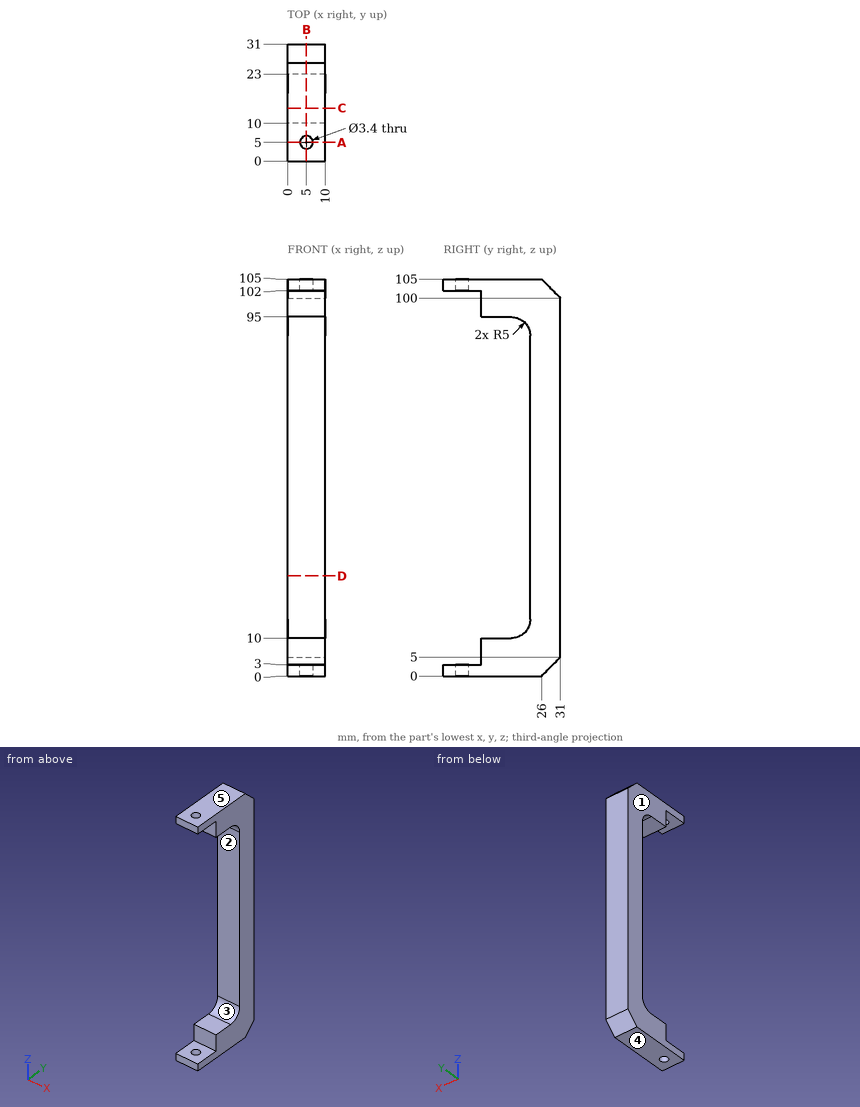
Print and shaded views of the part. All mm, measured from the part's lowest x, y and z. A direction names the side the tool comes from. Coordinates: 2 decimals unless noted, no trailing zeros. Write each loop counter-clockwise with the first axis right and the second up, starting at its lowest first coordinate (ties: lowest second). Pieces come first, ordered by that corner, then holes.
(1) Drill centre lines: probe 1 along Z at (x, y) = (8.25, 17.5); probe 2 along Z at (x, y) = (5.25, 1); probe 3 along Y at (x, z) = (9.25, 87.5). Where is each one in solid material? Low to high.
(2) Cut at C-C, the plane y = 14. List the corners of the cut face in (x, z), and give its area (3 significant figures).
(3) Cut at B-B, the plane x = 5. List the corners of the cut face in (y, z), and give its area (3 significant figures).
(4) 3-axis set-ups, long thin cutter, end or side, ignore diameter. For the marked faces 1 and 2: which of +Z, -Z, +X, -X, +Y, -Y reach the whole face in a straight line?
(5) Cut at A-A, the plane y = 5. List the corners of the cut face in (x, z), and give its area (3 significant figures).
(6) Flat gauge pins, fed straight in: pin 1 (3 mm diameter, centred on x = 2, z = 46.5, fed in from -Y); pin 2 (2.5 mm diameter, centred on x = 5, y = 5, fed in from -Z); pin 3 (5.5 mm diameter, centred on x = 2.5, z = 98, fed in from -Y). Where does each tip first touch, or does it go through?
(7) Cut at D-D, the plane z = 26.5. List the corners of the cut face in (x, y), and give its area (3 significant figures).
(8) Two-plate mould, pull along Z, no slides. Class the marked faces 3, 4 and 5: +Z half, -Z half, draft (parallel to the pull), parting line (faces both ways), or undercut.
Geometry says:
1. probe 1: z = 0 to 10, 95 to 105
1. probe 2: z = 0 to 3, 102 to 105
1. probe 3: y = 23 to 31
2. outline: (0, 0) - (10, 0) - (10, 10) - (0, 10) - close; (0, 95) - (10, 95) - (10, 105) - (0, 105) - close
2. area: 200 mm2
3. outline: (0, 0) - (3.3, 0) - (3.3, 3) - (0, 3) - close; (0, 102) - (3.3, 102) - (3.3, 105) - (0, 105) - close; (6.7, 0) - (26, 0) - (31, 5) - (31, 100) - (26, 105) - (6.7, 105) - (6.7, 102) - (10, 102) - (10, 95) - (18, 95) arc R5 cw to (23, 90) - (23, 15) arc R5 cw to (18, 10) - (10, 10) - (10, 3) - (6.7, 3) - close
3. area: 1,130 mm2
4. face 1: +Z, -Z, -X, +Y, -Y
4. face 2: +X, -X, -Y
5. outline: (0, 0) - (3.3, 0) - (3.3, 3) - (0, 3) - close; (0, 102) - (3.3, 102) - (3.3, 105) - (0, 105) - close; (6.7, 0) - (10, 0) - (10, 3) - (6.7, 3) - close; (6.7, 102) - (10, 102) - (10, 105) - (6.7, 105) - close
5. area: 39.6 mm2
6. pin 1: stops at y = 23
6. pin 2: passes through
6. pin 3: stops at y = 10
7. outline: (0, 23) - (10, 23) - (10, 31) - (0, 31) - close
7. area: 80.0 mm2
8. face 3: undercut
8. face 4: -Z half
8. face 5: +Z half
